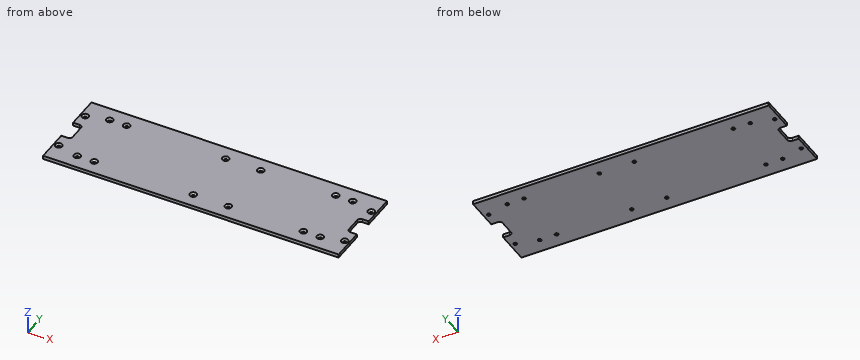
from build123d import *

# Parameters (mm, degrees)
BOSS_EXTRU_1_DEPTH                             = 3.175
FRAISAGE_POUR_VIS_T_TE_FRAIS_E_M31_D           = 3.2
FRAISAGE_POUR_VIS_T_TE_FRAIS_E_M31_CSINK_D     = 6.3
FRAISAGE_POUR_VIS_T_TE_FRAIS_E_M31_CSINK_ANGLE = 90
FRAISAGE_POUR_VIS_T_TE_FRAIS_E_M32_D           = 3.2
FRAISAGE_POUR_VIS_T_TE_FRAIS_E_M32_CSINK_D     = 6.3
FRAISAGE_POUR_VIS_T_TE_FRAIS_E_M32_CSINK_ANGLE = 90
CONG_1_R                                       = 3


with BuildPart() as part:
    # Esquisse1 → Boss.-Extru.1 (new body)
    with BuildSketch(Plane.XY):
        Polygon((-262.5, 10), (-262.5, 41), (13, 41), (13, 10), (4, 10), (4, -10), (13, -10), (13, -41), (-262.5, -41), (-262.5, -10), (-253.5, -10), (-253.5, 10), align=None)
    extrude(amount=BOSS_EXTRU_1_DEPTH)

    # Fraisage pour vis à tête fraisée M31 (through all)
    with Locations(Plane.XY.offset(3.175)):
        with Locations((-11.515, 27.5), (-11.515, -27.5), (-237.985, -27.5), (-237.985, 27.5), (-27.25, 27.5), (-27.25, -27.5), (-222.25, -27.5), (-222.25, 27.5), (-97.25, 27.5), (-97.25, -27.5), (-129.905, 27.5), (-129.905, -27.5)):
            CounterSinkHole(FRAISAGE_POUR_VIS_T_TE_FRAIS_E_M31_D / 2, FRAISAGE_POUR_VIS_T_TE_FRAIS_E_M31_CSINK_D / 2, counter_sink_angle=FRAISAGE_POUR_VIS_T_TE_FRAIS_E_M31_CSINK_ANGLE)

    # Fraisage pour vis à tête fraisée M32 (through all)
    with Locations(Plane.XY.offset(3.175)):
        with Locations((8.5, -22.5), (8.5, 22.5), (-258, -22.5), (-258, 22.5)):
            CounterSinkHole(FRAISAGE_POUR_VIS_T_TE_FRAIS_E_M32_D / 2, FRAISAGE_POUR_VIS_T_TE_FRAIS_E_M32_CSINK_D / 2, counter_sink_angle=FRAISAGE_POUR_VIS_T_TE_FRAIS_E_M32_CSINK_ANGLE)

    # Congé1
    cong_1_edges = [part.edges().sort_by_distance(p)[0] for p in [
        (-253.5, -10, 1.5875),
        (-253.5, 10, 1.5875),
        (4, 10, 1.5875),
        (4, -10, 1.5875),
    ]]
    fillet(cong_1_edges, radius=CONG_1_R)


solid = part.part
Model file for the job. Use its own axes, mm. Round coordinates to 2 decimals unless told otherwise and drop trailing zeros. Write each question's results on one line, items separated by ' | '. Start each with the question number.
(1) Probe probe 1 along Y at (x, z) = (-258, 0.75); probe 2 along X at (y, z) = (22.5, 0.85); probe 3 along X at (y, z) = (-1.5, 2.05). List the from-to ranges inside material, lowest first. Write a range as from..to.
(2) Drop flat-ended pins along their axis: pin 1 (1.9 mm diameter, centred on x = 8.5, y = 22.5, fed in from -Z); pin 2 (5 mm diameter, centred on x = -11.515, y = -27.5, fed in from +Z) (3 decimals); pin 3 (1 mm diameter, centred on y = -4.5, z = 2, fed in from +X). Give the stop position or say it passes through.
(3) Saw through at A-A, the plane z = 0.55. State how many separate pieces and enclosed holes the cut face has, then the cut area to 3 significant figures.
Established:
1) probe 1: y = -41..-24.1, -20.9..-10, 10..20.9, 24.1..41 | probe 2: x = -262.5..-259.6, -256.4..6.9, 10.1..13 | probe 3: x = -253.5..4
2) pin 1: passes through | pin 2: stops at z = 2.525 | pin 3: stops at x = 4
3) separate pieces: 1 | enclosed holes: 16 | area: 22,100 mm^2
